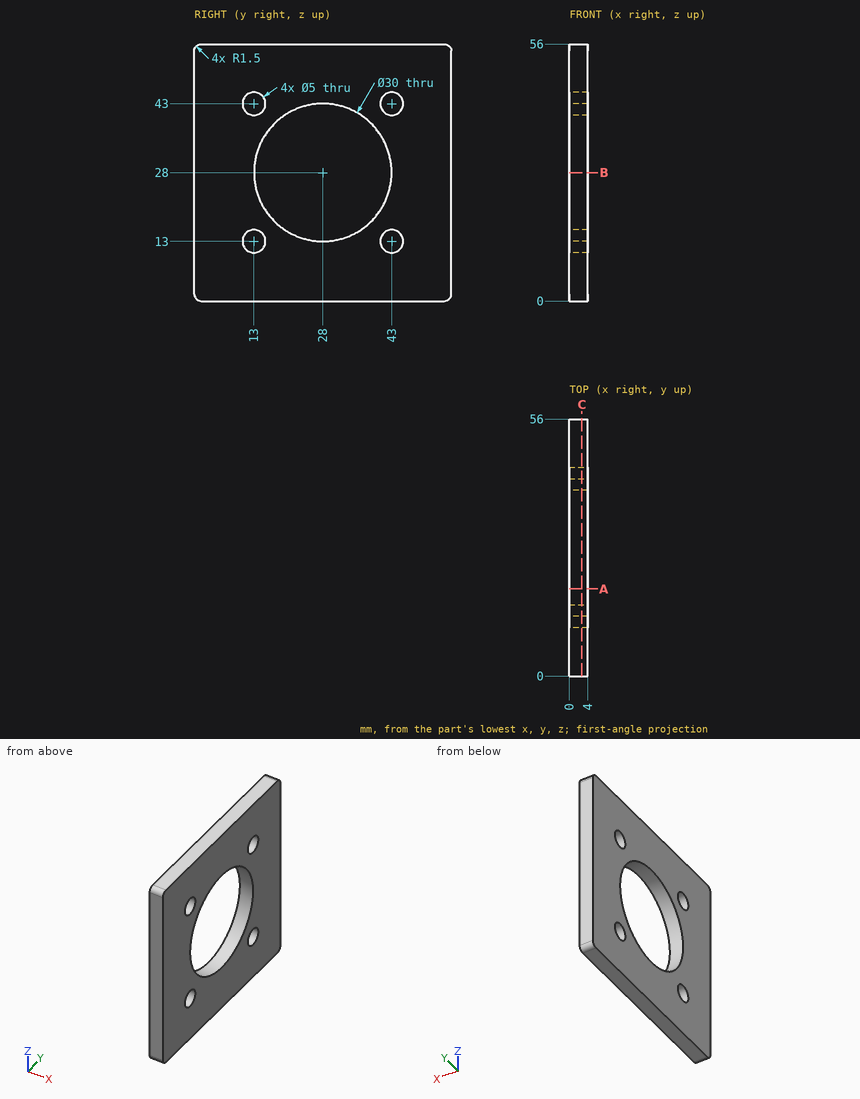
Check sheet for the drawn part. Datum: minimum x, y, z corner. Units: mm. Round coordinates to 2 decimals unless told otherwise and drop trailing zeros. Write each loop counter-clockwise with the first axis right and the second up, starting at its lowest first coordinate (ties: lowest second). Pieces come first, ordered by that corner, then holes. Notation, with made-up numbers: (81, 64) -> (117, 64) arc R8 cw to (117, 69) -> close; hole circle Ø1 at (-6, 54). An arc over 180 degrees is marked (long way). Write each question's results on one line, items separated by ' | '.
Q1. Sectioned sample at B-B, the plane z = 28. Record the boundary of the cut face in (x, y), and give its area (3 significant figures).
Derived:
outline: (0, 0) -> (4, 0) -> (4, 13) -> (0, 13) -> close; (0, 43) -> (4, 43) -> (4, 56) -> (0, 56) -> close | area: 104 mm²
Q2. Sectioned sample at A-A, the plane y = 19. Record the boundary of the cut face in (x, z), and give its area (3 significant figures).
Derived:
outline: (0, 0) -> (4, 0) -> (4, 16) -> (0, 16) -> close; (0, 40) -> (4, 40) -> (4, 56) -> (0, 56) -> close | area: 128 mm²
Q3. Sectioned sample at C-C, the plane x = 2.75. Record the boundary of the cut face in (y, z).
Derived:
outline: (0, 1.5) arc R1.5 ccw to (1.5, 0) -> (54.5, 0) arc R1.5 ccw to (56, 1.5) -> (56, 54.5) arc R1.5 ccw to (54.5, 56) -> (1.5, 56) arc R1.5 ccw to (0, 54.5) -> close; hole circle Ø5 at (13, 13); hole circle Ø5 at (13, 43); hole circle Ø30 at (28, 28); hole circle Ø5 at (43, 13); hole circle Ø5 at (43, 43)
Q4. Go/stop test with a flat-tipped pin: pin 1 Ø4.5 at (y, z) = (13, 13) entering from -X. Record where the tip stops, or that it passes through.
Derived:
pin 1: passes through
Q5. Thickness scan on probe 1 along Z at (x, y) = (2.8, 28); probe 2 along Z at (x, y) = (1, 45); probe 3 along Z at (x, y) = (0.2, 29.5). Record the ranges inside material, lowest first.
Derived:
probe 1: z = 0 to 13, 43 to 56 | probe 2: z = 0 to 11.5, 14.5 to 41.5, 44.5 to 56 | probe 3: z = 0 to 13.08, 42.92 to 56
